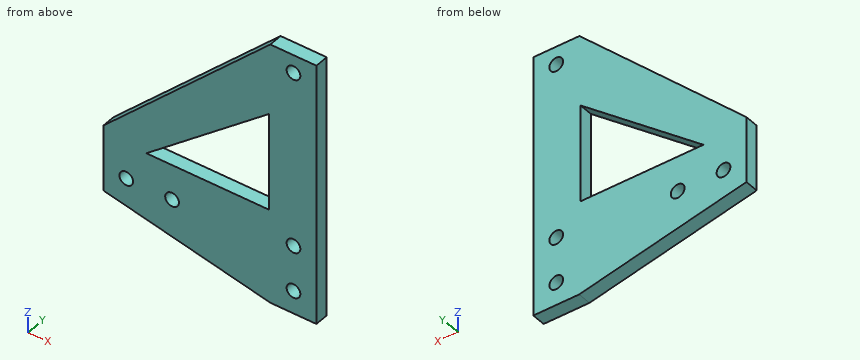
```python
from build123d import *

# Parameters (mm, degrees)
SKETCH1_R           = 1.5
BOSS_EXTRUDE1_DEPTH = 3
SKETCH4_R           = 1.5
CUT_EXTRUDE2_DEPTH  = 7
SKETCH5_W           = 46.5
SKETCH5_H           = 2
CUT_EXTRUDE3_DEPTH  = 7
CUT_EXTRUDE4_DEPTH  = 7
CUT_EXTRUDE5_DEPTH  = 7


with BuildPart() as part:
    # Sketch1 → Boss-Extrude1 (new body)
    with BuildSketch(Plane(origin=(0, 0, 0), x_dir=(1, 0, 0), z_dir=(0, 1, 0))):
        Polygon((5, 16.666723622), (5, 56.73), (-5, 56.73), (-5, 5.234024539), (5, 5.234024539), (31.5, 5.234024539), (41.5, 5.234024539), (41.5, 64.6), (31.5, 64.6), (31.5, 54.48), (31.5, 16.666723622), align=None)
        with Locations((0, 10.18)):
            Circle(SKETCH1_R, mode=Mode.SUBTRACT)
        with Locations((36.5, 11.18)):
            Circle(SKETCH1_R, mode=Mode.SUBTRACT)
        with Locations((0, 51.73)):
            Circle(SKETCH1_R, mode=Mode.SUBTRACT)
        with Locations((36.5, 49.6)):
            Circle(SKETCH1_R, mode=Mode.SUBTRACT)
        with Locations((36.5, 59.6)):
            Circle(SKETCH1_R, mode=Mode.SUBTRACT)
        Polygon((-5, 56.73), (5, 56.73), (31.5, 54.48), (31.5, 64.6), align=None)
        Polygon((31.5, 54.48), (5, 56.73), (5, 16.666723622), (31.5, 16.666723622), align=None)
    extrude(amount=BOSS_EXTRUDE1_DEPTH)

    # Sketch4 → Cut-Extrude2 (cut)
    with BuildSketch(Plane(origin=(0, 3, 0), x_dir=(1, 0, 0), z_dir=(0, 1, 0))):
        with Locations((10, 51.73)):
            Circle(SKETCH4_R)
    extrude(amount=-CUT_EXTRUDE2_DEPTH, mode=Mode.SUBTRACT)

    # Sketch5 → Cut-Extrude3 (cut)
    with BuildSketch(Plane(origin=(0, 3, 0), x_dir=(1, 0, 0), z_dir=(0, 1, 0))):
        with Locations((18.25, 6.234024539)):
            Rectangle(SKETCH5_W, SKETCH5_H)
    extrude(amount=-CUT_EXTRUDE3_DEPTH, mode=Mode.SUBTRACT)

    # Sketch6 → Cut-Extrude4 (cut)
    with BuildSketch(Plane(origin=(0, 3, 0), x_dir=(1, 0, 0), z_dir=(0, 1, 0))):
        Polygon((31.443621834, 7.234024539), (-5, 42.312799573), (-5, 7.234024539), align=None)
    extrude(amount=-CUT_EXTRUDE4_DEPTH, mode=Mode.SUBTRACT)

    # Sketch7 → Cut-Extrude5 (cut)
    with BuildSketch(Plane(origin=(0, 3, 0), x_dir=(1, 0, 0), z_dir=(0, 1, 0))):
        Polygon((31.193110027, 22.772878628), (31.193110027, 44.066382221), (4.388346681, 44.066382221), align=None)
    extrude(amount=-CUT_EXTRUDE5_DEPTH, mode=Mode.SUBTRACT)


solid = part.part
```
Check sheet for the modelled part. Datum: model origin and axes. Units: mm. Coordinates: 2 decimals unless noted, no trailing zeros. Order: outer loops, then holes, each group sorted by start corner. A loop starts at its lowest first (then second) coordinate and runs counter-clockwise, first axis right, second up. Notation, with made-up numbers: M 16,23 L 48,23 A10 ccw 48,39 Z; hole C 76,21.25 d4. An arc over 180 degrees is marked long. Write each question's results on one line, items separated by ' | '. Start each with the question number.
1. Material ranges on probe 1 along Z at (x, y) = (36.5, 1.4); probe 2 along X at (y, z) = (2.15, -49.6); probe 3 along Z at (x, y) = (37.5, 0.85), recorded low to high.
2. Cross-section at B-B on z = -49.6. Record the cut outline in (x, y), and give its area (4 significant figures).
3. Cross-section at A-A on x = 36.5. Record the cut outline in (y, z), and give its area (3 significant figures).
4. Go/stop test with flat-tipped pins: P1, Ø2.5, axis at x = 36.5, z = -11.18, coming from the -Y side; P2, Ø1.5, axis at y = 1, z = -37, coming from the -X side. Record where each tip stops, or that it passes through.
5. Cross-section at C-C on y = 2.15. Record the cut outline in (x, z).
6. Cross-section at D-D on x = 10. Record the cut outline in (y, z).
Checks:
1) probe 1: z = -64.6 to -61.1, -58.1 to -51.1, -48.1 to -12.68, -9.68 to -7.23 | probe 2: x = -5 to 35, 38 to 41.5 | probe 3: z = -64.6 to -60.72, -58.48 to -50.72, -48.48 to -12.3, -10.06 to -7.23
2) outline: M -5,0 L 35,0 L 35,3 L -5,3 Z; M 38,0 L 41.5,0 L 41.5,3 L 38,3 Z | area: 130.5 mm²
3) outline: M 0,-64.6 L 3,-64.6 L 3,-61.1 L 0,-61.1 Z; M 0,-58.1 L 3,-58.1 L 3,-51.1 L 0,-51.1 Z; M 0,-48.1 L 3,-48.1 L 3,-12.68 L 0,-12.68 Z; M 0,-9.68 L 3,-9.68 L 3,-7.23 L 0,-7.23 Z | area: 145 mm²
4) P1: passes through | P2: stops at x = -0.26
5) outline: M -5,-56.73 L 31.5,-64.6 L 41.5,-64.6 L 41.5,-7.23 L 31.44,-7.23 L -5,-42.31 Z; hole C 0,-51.73 d3; hole M 4.39,-44.07 L 31.19,-44.07 L 31.19,-22.77 Z; hole C 10,-51.73 d3; hole C 36.5,-59.6 d3; hole C 36.5,-49.6 d3; hole C 36.5,-11.18 d3
6) outline: M 0,-59.96 L 3,-59.96 L 3,-53.23 L 0,-53.23 Z; M 0,-50.23 L 3,-50.23 L 3,-44.07 L 0,-44.07 Z; M 0,-39.61 L 3,-39.61 L 3,-27.87 L 0,-27.87 Z
